Geometry check sheet. Reference: the model listing, model coordinates, mm. A direction names the side the tool comes from. Coordinates: 2 decimals unless noted, no trailing zeros. Order: outer loops, then holes, each group sorted by start corner. A loop starts at its lowest first (then second) coordinate and runs counter-clockwise, first axis right, second up. Notation, with made-up numbers: (48.5, -1) -> (103.5, -1) arc R22 cw to (103.5, 32) -> close; hole circle Ø8 at (4.25, -10). An arc over 180 degrees is marked (long way). Answer as CSV lines item,"result". Start each with the question number.
from build123d import *

# Parameters (mm, degrees)
CASING_W            = 8.3
CASING_H            = 7.392304845
BOSS_EXTRUDE2_DEPTH = 65
SKETCH10_W          = 10.3
SKETCH10_H          = 7.392395682
TOP_CUT_DEPTH       = 16.35
SKETCH11_W          = 10.3
SKETCH11_H          = 7.40522356
BOT_CUT_DEPTH       = 16.35
SKETCH13_W          = 8.3
SKETCH13_H          = 30.255654569
CUT_EXTRUDE8_DEPTH  = 68.55767906
FILLET1_R           = 1
FILLET2_R           = 2


with BuildPart() as part:
    # Casing → Boss-Extrude2 (new body)
    # profile 1 of 2: a face of its own
    with BuildSketch(Plane.XY):
        Polygon((-9.2, 0), (9.2, 0), (10.066025404, 1.5), (8.333974596, 1.5), (5.15, 1.5), (5.15, 8.892304845), (12.601923789, 8.892304845), (14.333974596, 8.892304845), (15.2, 10.392304845), (-15.2, 10.392304845), (-14.333974596, 8.892304845), (-12.601923789, 8.892304845), (-5.15, 8.892304845), (-5.15, 1.5), (-8.333974596, 1.5), (-10.066025404, 1.5), align=None)
        with Locations((0, 5.196152422)):
            Rectangle(CASING_W, CASING_H, mode=Mode.SUBTRACT)
    # profile 2 of 2: a face of its own
    with BuildSketch(Plane.XY):
        with Locations((0, 5.196152422)):
            Rectangle(CASING_W, CASING_H)
    extrude(amount=BOSS_EXTRUDE2_DEPTH)

    # Sketch10 → Top_Cut (cut)
    with BuildSketch(Plane.XY.offset(65)):
        with Locations((0, 5.196197841)):
            Rectangle(SKETCH10_W, SKETCH10_H)
    extrude(amount=-TOP_CUT_DEPTH, mode=Mode.SUBTRACT)

    # Sketch11 → Bot_Cut (cut)
    with BuildSketch(Plane(origin=(0, 0, 0), x_dir=(-1, 0, 0), z_dir=(0, 0, -1))):
        with Locations((0, 5.20261178)):
            Rectangle(SKETCH11_W, SKETCH11_H)
    extrude(amount=-BOT_CUT_DEPTH, mode=Mode.SUBTRACT)

    # Sketch13 → Cut-Extrude8 (cut, through all)
    with BuildSketch(Plane(origin=(0, 10.392304845, 0), x_dir=(1, 0, 0), z_dir=(0, 1, 0))):
        with Locations((0, -32.477827285)):
            Rectangle(SKETCH13_W, SKETCH13_H)
    extrude(amount=-CUT_EXTRUDE8_DEPTH, mode=Mode.SUBTRACT)

    # Fillet1
    fillet1_edges = [part.edges().sort_by_distance(p)[0] for p in [
        (-5.15, 5.196152423, 48.65),
        (5.15, 5.196152423, 48.65),
        (5.15, 5.196152423, 16.35),
        (-5.15, 5.196152423, 16.35),
    ]]
    fillet(fillet1_edges, radius=FILLET1_R)

    # Fillet2
    fillet2_edges = [part.edges().sort_by_distance(p)[0] for p in [
        (4.15, 10.392304845, 32.477827285),
        (-4.15, 10.392304845, 32.477827285),
    ]]
    fillet(fillet2_edges, radius=FILLET2_R)


solid = part.part
Q1. Thickness scan on L1, parallel to Y at x = 7, z = 44; L2, parallel to Z at x = 0, y = 2.5; L3, parallel to X at y = 7.25, z = 32. Record the ranges inside material, lowest first.
Q2. Access from +Z, -Z, +X, -X, +Y, -Y to the whole of each face (thin tool, end or side, straight path). Record for faces 4 (the flat face through (4.15, 4, 33)), 5 (the cylindrical face through (4.72, 9.79, 32.27)), 6 (the flat face through (0, 8.892, 57)).
Q3. Release check for a two-part mould opening along Z. For faces 1 (the flat face through (7, 10.392, 32)), 2 (the flat face through (0, 10, 0)), 3 (the flat face through (0, 5, 17.35)) record: released by +Z, released by -Z, zero draft, split by the parting line, or undercut.
Q4. Go/stop test with flat-tipped pins: pin 1 Ø3 at (x, z) = (-3.5, 29.5) entering from +Y; pin 2 Ø4 at (y, z) = (4, 26) entering from -X; pin 3 Ø3.5 at (x, y) = (0, 6.5) entering from -Z. Record where each tip stops, or that it passes through.
Q5. Sectioned sample at C-C, the plane x = 0.5. Record the cut outline in (y, z).
Q6. Sectioned sample at B-B, the plane z = 29.5. Record the cut outline in (x, y), then the cut area to 3 significant figures.
Q7. Sectioned sample at A-A, the plane y = 2.25. Record the cut outline in (x, z).
Geometry results:
1,L1,"y = 0 to 1.5, 8.89 to 10.39"
1,L2,"z = 16.35 to 17.35, 47.61 to 48.65"
1,L3,"x = -5.15 to -4.15, 4.15 to 5.15"
2,face 4,"+Y, -Y"
2,face 5,"+Y"
2,face 6,"+Z, +X, -X"
3,face 1,"zero draft"
3,face 2,"released by -Z"
3,face 3,"undercut"
4,pin 1,"stops at y = 10.03"
4,pin 2,"stops at x = -5.15"
4,pin 3,"stops at z = 16.35"
5,outline,"(0, 0) -> (1.5, 0) -> (1.5, 16.35) -> (8.91, 16.35) -> (8.91, 0) -> (10.39, 0) -> (10.39, 17.35) -> (0, 17.35) -> close; (0, 47.61) -> (10.39, 47.61) -> (10.39, 65) -> (8.89, 65) -> (8.89, 48.65) -> (1.5, 48.65) -> (1.5, 65) -> (0, 65) -> close"
6,outline,"(-15.2, 10.39) -> (-14.33, 8.89) -> (-5.15, 8.89) -> (-5.15, 1.5) -> (-10.07, 1.5) -> (-9.2, 0) -> (-4.15, 0) -> (-4.15, 8.39) arc R2 ccw to (-6.15, 10.39) -> close; (4.15, 0) -> (9.2, 0) -> (10.07, 1.5) -> (5.15, 1.5) -> (5.15, 8.89) -> (14.33, 8.89) -> (15.2, 10.39) -> (6.15, 10.39) arc R2 ccw to (4.15, 8.39) -> close"
6,area,"61.4 mm^2"
7,outline,"(-5.15, 17.35) arc R1 ccw to (-4.15, 16.35) -> (4.15, 16.35) arc R1 ccw to (5.15, 17.35) -> (5.15, 47.65) arc R1 ccw to (4.15, 48.65) -> (-4.15, 48.65) arc R1 ccw to (-5.15, 47.65) -> close; hole (-4.15, 17.35) -> (4.15, 17.35) -> (4.15, 47.61) -> (-4.15, 47.61) -> close"
